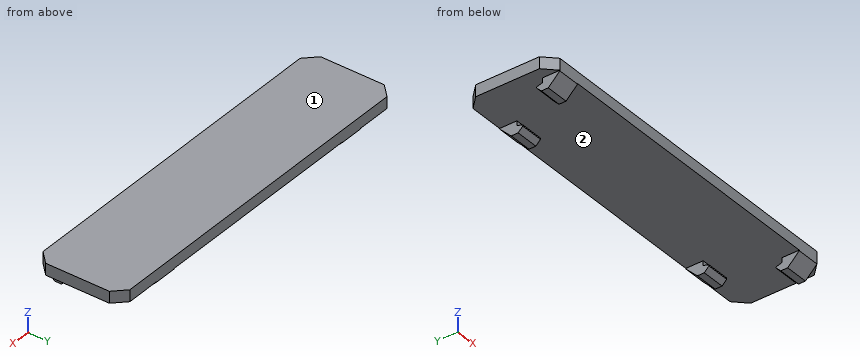
from build123d import *

# Parameters (mm, degrees)
F0_W     = 62
F0_H     = 15
F1_DEPTH = 2
F2_W     = 4
F2_H     = 3
F3_DEPTH = 2.1
F4_SIZE  = 2
F5_DEPTH = 1
F7_DEPTH = 70
F10_SIZE = 0.8


with BuildPart() as f1:
    # F0 (on Top) → F1 (new body)
    with BuildSketch(Plane.XY):
        Rectangle(F0_W, F0_H)
    extrude(amount=F1_DEPTH)

    # F2 (on face) → F3 (join)
    with BuildSketch(Plane(origin=(0, 0, 0), x_dir=(1, 0, 0), z_dir=(0, 0, -1))):
        with Locations((-27, 6)):
            Rectangle(F2_W, F2_H)
        with Locations((-21, -6)):
            Rectangle(F2_W, F2_H)
        with Locations((21, -6)):
            Rectangle(F2_W, F2_H)
        with Locations((27, 6)):
            Rectangle(F2_W, F2_H)
    extrude(amount=F3_DEPTH)

    # F4
    f4_edges = [f1.edges().sort_by_distance(p)[0] for p in [
        (-31, -7.5, 1),
        (-31, 7.5, 1),
        (-21, 7.5, -2.1),
        (-27, -7.5, -2.1),
        (31, -7.5, 1),
        (27, -7.5, -2.1),
        (31, 7.5, 1),
        (21, 7.5, -2.1),
    ]]
    chamfer(f4_edges, length=F4_SIZE)

    # F5 (add, symmetric): faces of the model
    f5_faces = [f1.faces().sort_by_distance(p)[0] for p in [
        (-27, -4.5, -1.05),
        (27, -4.5, -1.05),
        (21, 4.5, -1.05),
        (-21, 4.5, -1.05),
    ]]
    extrude(f5_faces, amount=F5_DEPTH, both=True, dir=(0, 1, 0))


with BuildPart() as f7:
    # F6 (on face) → F7 (new body)
    with BuildSketch(Plane(origin=(-29, 0, 0), x_dir=(0, -1, 0), z_dir=(-1, 0, 0))):
        Polygon((4.5, 0), (3.5, 0), (3.5, -1.1), (4.5, -0.8), align=None)
    extrude(amount=-F7_DEPTH)


with BuildPart() as f8_1:
    # F8: instance of F7
    add(f7.part.mirror(Plane.XZ))


with BuildPart() as f1_1:
    add(f1.part)

    # F9: cut F7, F8_1
    add(f7.part, mode=Mode.SUBTRACT)
    add(f8_1.part, mode=Mode.SUBTRACT)

    # F10
    f10_edges = [f1_1.edges().sort_by_distance(p)[0] for p in [
        (-27, -3.5, -2.1),
        (27, -3.5, -2.1),
        (21, 3.5, -2.1),
        (-21, 3.5, -2.1),
    ]]
    chamfer(f10_edges, length=F10_SIZE)


solid = f1_1.part
Can you work these out from the model? Positions are in its coordinate system, mm. Face numbers are marked on the shaded views. Give positions to 0.01 mm unless a question says otherwise; leave off trailing zeros. Order: outer loops, then holes, each group sorted by start corner. A loop starts at its lowest first (then second) coordinate and runs counter-clockwise, first axis right, second up. Notation, with made-up numbers: M 59,66.25 L 86,66.25 A22 cw 86,96.25 Z; hole C 15.25,35 d6. An arc over 180 degrees is marked long. One line per item, written item: value.
Item 1: For pin 1 (1.7 mm diameter, centred on y = 5.5, z = -1, fed in from -X); pin 2 (1.1 mm diameter, centred on y = -5.5, z = -1, fed in from +X); pin 3 (4 mm diameter, centred on x = -22.5, y = -3.5, fed in from -Z), each with a flat end and sliding along its axis, tell me the tip position at first contact or that it passes through.
Verdict:
pin 1: x = -23
pin 2: x = 29
pin 3: z = 0
Item 2: If we section it at A-A on x = -26: Write out the boundary of the cut face in (y, z).
Verdict:
outline: M -7.5,-0.1 L -5.5,-2.1 L -4.3,-2.1 L -3.5,-1.3 L -3.5,-1.1 L -4.5,-0.8 L -4.5,0 L 7.5,0 L 7.5,2 L -7.5,2 Z
Item 3: Please list where these lines run through material, in increasing order: line 1 (X direction, y = 5.25, z = -1.6); line 2 (Z direction, x = -9.5, y = -2.5); line 3 (X direction, y = -6.25, z = 1.8).
Verdict:
line 1: -23 to -19, 19 to 23
line 2: 0 to 2
line 3: -30.25 to 30.25
Item 4: If we section it at C-C on x = 13.5: Write out the boundary of the cut face in (y, z), and give its area (3 significant figures).
Verdict:
outline: M -7.5,0 L 7.5,0 L 7.5,2 L -7.5,2 Z
area: 30.0 mm2
Item 5: If we mould it in two halves opening along X, with no side actions, what happens to the marked faces 1 and 2? For each: pulls with the +X half, pulls with the -X half, needs draft (parallel to the pull), parting line crosses it, or undercut.
Verdict:
face 1: needs draft
face 2: undercut
Item 6: If we section it at B-B on y = -2.25: Write out the boundary of the cut face in (x, z).
Verdict:
outline: M -31,0 L 31,0 L 31,2 L -31,2 Z
